```python
from build123d import *

# Parameters (mm, degrees)
SKETCH1_R                              = 19.05
F_1_5_DIAMETER_2_TALL_CYLINDER_DEPTH   = 50.8
SKETCH2_R                              = 19.05
SKETCH2_R_2                            = 15.875
F_1_25_DIAMETER_X_5_CYLINDER_CUT_DEPTH = 12.7
SKETCH3_R                              = 11.1125
CUT_EXTRUDE2_DEPTH                     = 6.35
SKETCH4_W                              = 9.525
SKETCH4_H                              = 38.1
CUT_EXTRUDE3_DEPTH                     = 9.525
SKETCH5_W                              = 38.1
SKETCH5_H                              = 6.4008
CUT_EXTRUDE4_DEPTH                     = 6.35
SKETCH11_R                             = 9.525
CUT_EXTRUDE5_DEPTH                     = 6.35
SKETCH12_W                             = 6.4008
SKETCH12_H                             = 19.05
CUT_EXTRUDE6_DEPTH                     = 6.35
SKETCH13_W                             = 38.1
SKETCH13_H                             = 22.225
CUT_EXTRUDE7_DEPTH                     = 6.35


with BuildPart() as part:
    # Sketch1 → 1.5" diameter 2" tall cylinder (new body)
    with BuildSketch(Plane(origin=(0, 0, 0), x_dir=(1, 0, 0), z_dir=(0, 1, 0))):
        Circle(SKETCH1_R)
    extrude(amount=F_1_5_DIAMETER_2_TALL_CYLINDER_DEPTH)

    # Sketch2 → 1.25" diameter x .5" cylinder cut (cut)
    with BuildSketch(Plane(origin=(0, 50.8, 0), x_dir=(1, 0, 0), z_dir=(0, 1, 0))):
        Circle(SKETCH2_R)
        Circle(SKETCH2_R_2, mode=Mode.SUBTRACT)
    extrude(amount=-F_1_25_DIAMETER_X_5_CYLINDER_CUT_DEPTH, mode=Mode.SUBTRACT)

    # Sketch3 → Cut-Extrude2 (cut)
    with BuildSketch(Plane(origin=(0, 50.8, 0), x_dir=(1, 0, 0), z_dir=(0, 1, 0))):
        Circle(SKETCH3_R)
    extrude(amount=-CUT_EXTRUDE2_DEPTH, mode=Mode.SUBTRACT)

    # Sketch4 → Cut-Extrude3 (cut)
    with BuildSketch(Plane(origin=(0, 50.8, 0), x_dir=(1, 0, 0), z_dir=(0, 1, 0))):
        Rectangle(SKETCH4_W, SKETCH4_H)
    extrude(amount=-CUT_EXTRUDE3_DEPTH, mode=Mode.SUBTRACT)

    # Sketch5 → Cut-Extrude4 (cut)
    with BuildSketch(Plane(origin=(0, 50.8, 0), x_dir=(1, 0, 0), z_dir=(0, 1, 0))):
        Rectangle(SKETCH5_W, SKETCH5_H)
    extrude(amount=-CUT_EXTRUDE4_DEPTH, mode=Mode.SUBTRACT)

    # Sketch11 → Cut-Extrude5 (cut)
    with BuildSketch(Plane(origin=(0, 0, 0), x_dir=(-1, 0, 0), z_dir=(0, -1, 0))):
        Circle(SKETCH11_R)
    extrude(amount=-CUT_EXTRUDE5_DEPTH, mode=Mode.SUBTRACT)

    # Sketch12 → Cut-Extrude6 (cut)
    with BuildSketch(Plane.XZ):
        with Locations((0, -9.525)):
            Rectangle(SKETCH12_W, SKETCH12_H)
    extrude(amount=-CUT_EXTRUDE6_DEPTH, mode=Mode.SUBTRACT)

    # Sketch13 → Cut-Extrude7 (cut)
    with BuildSketch(Plane.XZ):
        with Locations((0, 7.9375)):
            Rectangle(SKETCH13_W, SKETCH13_H)
    extrude(amount=-CUT_EXTRUDE7_DEPTH, mode=Mode.SUBTRACT)


solid = part.part
```
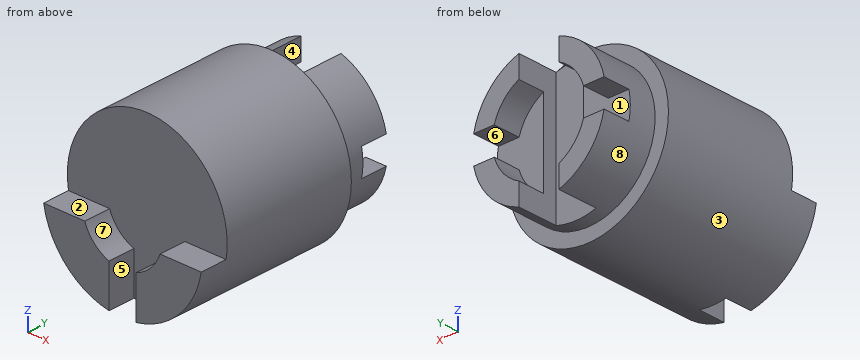
Geometry: final body of the model. Coordinates: model frame, mm. Face numbers are marked on the shaded views. A direction names the side the tool comes from. Coordinates: 2 decimals unless noted, no trailing zeros. Order: outer loops, then holes, each group sorted by start corner. A loop starts at its lowest first (then second) coordinate and runs counter-clockwise, first axis right, second up. Notation, with made-up numbers: (-8, 71) - (0, 71) arc R10 cw to (0, 77) - close; hole circle Ø2 at (84, -10). An arc over 180 degrees is marked (long way). Return JSON: item names as keys, results as strings. Group by question number.
1. Material intervals for line 1 along Y through (x, z) = (-1, -13) (3 decimals); line 2 along Y through (x, z) = (-11.5, 4); line 3 along X through (y, z) = (44, -4), sorted ascending. Write a range as [from, to].
2. Pin query (flat end, axial travel): pin 1 (5 mm diameter, centred on x = 14, y = 14, fed in from +Z); pin 2 (12 mm diameter, centred on x = 8, y = 16, fed in from +Z); pin 3 (3 mm diameter, centred on x = 9.5, y = 14, fed in from +Z). Return the tip coordinate at first contact, or that it passes through.
3. Pull-direction query (X, two-part tool) for the marked faces 1, 2 and 3; classes: pulls with the +X half, pulls with the -X half, needs draft (parallel to the pull), parting line crosses it, or undercut.
4. Cut plane D-D (x = -14.5). Output: boundary loops of the cut face in (y, z) (3 decimals).
5. Set-up query: the marked faces 4, 5, 6, 7 and 8. Return all of +Z, -Z, +X, -X, +Y, -Y with unobstructed straight access to the full face (end or side cutting, diameter ignored); none if empty.
6. Cut plane C-C (y = 24). Output: boundary loops of the cut face in (x, z), plus the area to 3 significant figures.
7. Cut plane B-B (x = 0). Output: boundary loops of the cut face in (y, z) (3 decimals), plus the area to 3 significant figures.
Resolved:
{
 "1": {"line 1": "y = [6.35, 41.275]", "line 2": "y = [6.35, 50.8]", "line 3": "x = [-15.36, -4.76], [4.76, 15.36]"},
 "2": {"pin 1": "stops at z = 15.19", "pin 2": "stops at z = 18.94", "pin 3": "stops at z = 17.29"},
 "3": {"face 1": "undercut", "face 2": "needs draft", "face 3": "parting line crosses it"},
 "4": {"outline": "(0, -12.355) - (38.1, -12.355) - (38.1, -6.463) - (50.8, -6.463) - (50.8, -3.2) - (44.45, -3.2) - (44.45, 3.2) - (50.8, 3.2) - (50.8, 6.463) - (38.1, 6.463) - (38.1, 12.355) - (6.35, 12.355) - (6.35, -3.175) - (0, -3.175) - close"},
 "5": {"face 4": "+Z, -Z, +Y", "face 5": "+Z, -Z, -Y", "face 6": "+X, -X, +Y", "face 7": "+Z, -Y", "face 8": "+Y"},
 "6": {"outline": "circle Ø38.1 at (0, 0)", "area": "1,140 mm²"},
 "7": {"outline": "(6.35, -19.05) - (38.1, -19.05) - (38.1, -15.875) - (41.275, -15.875) - (41.275, 15.875) - (38.1, 15.875) - (38.1, 19.05) - (6.35, 19.05) - close", "area": "1,310 mm²"}
}
